from build123d import *

# Parameters (mm, degrees)
SKETCH009_W     = 7.72
SKETCH009_H     = 1
POCKET001_DEPTH = 26
POCKET002_DEPTH = 25


with BuildPart() as part:
    # Sketch008 → Revolution (revolve)
    with BuildSketch(Plane.XZ):
        Polygon((-1, 0), (-1, 3), (0, 3), (0, 2.5), (18.5, 2.5), (18.5, 3.2), (19.5, 2), (19.5, 0), align=None)
    revolve(axis=Axis((0, 0, 0), (1, 0, 0)))

    # Sketch009 → Pocket001 (cut)
    with BuildSketch(Plane.YZ):
        Rectangle(SKETCH009_W, SKETCH009_H)
    extrude(amount=POCKET001_DEPTH, mode=Mode.SUBTRACT)

    # Sketch010 → Pocket002 (cut, symmetric)
    with BuildSketch(Plane.XY):
        Polygon((15.1, 2.44949), (23.12, 2.44949), (23.12, -2.44949), (15.1, -2.44949), (15.1, -3.86051), (30.32, -3.86051), (30.32, 7.01949), (15.1, 7.01949), align=None)
    extrude(amount=POCKET002_DEPTH, both=True, mode=Mode.SUBTRACT)


with BuildPart() as part_1:
    # Body002 placement: moved
    add(part.part.moved(Location((-9.25, -10.5, 11.5))))


solid = part_1.part
Part model, mm, in its own coordinate system. A direction names the side the tool comes from. Round coordinates to 2 decimals unless told otherwise and drop trailing zeros. Order: outer loops, then holes, each group sorted by start corner. A loop starts at its lowest first (then second) coordinate and runs counter-clockwise, first axis right, second up. Notation, with made-up numbers: (-14.75, -19.75) -> (-10.75, -19.75) arc R33 ccw to (-10.75, 13.25) -> close; hole circle Ø1 at (-5, -13). An arc over 180 degrees is marked (long way). Put each result on its own line as item: value.
Q1. Band-saw the part on B-B (x = -7). Give the cut face in (y, z).
From the geometry:
outline: (-12.95, 11) arc R2.5 ccw to (-8.05, 11) -> close; (-12.95, 12) -> (-8.05, 12) arc R2.5 ccw to start
Q2. Band-saw the part on A-A (y = -10.5). Give the cut face in (x, z).
From the geometry:
outline: (-10.25, 8.5) -> (-9.25, 8.5) -> (-9.25, 9) -> (9.25, 9) -> (9.25, 8.3) -> (10.25, 9.5) -> (10.25, 11) -> (-9.25, 11) -> (-9.25, 12) -> (10.25, 12) -> (10.25, 13.5) -> (9.25, 14.7) -> (9.25, 14) -> (-9.25, 14) -> (-9.25, 14.5) -> (-10.25, 14.5) -> close
Q3. Pin check, flat tips, straight feed: pin 1 Ø1 at (y, z) = (-8, 13.5) entering from -X; pin 2 Ø1.5 at (x, y) = (4.5, -9) entering from +Z; pin 3 Ø0.6 at (x, z) = (9.5, 12.5) entering from +Y; pin 4 Ø0.6 at (x, z) = (9.5, 13) entering from -Y. Stop position of each tip, or through.
From the geometry:
pin 1: stops at x = -10.25
pin 2: stops at z = 13.88
pin 3: stops at y = -8.05
pin 4: stops at y = -12.95
Q4. Tool access for faces 1 (the face through (-9.25, -10.7, 11.5)), 2 (the face through (-9.7, -8.7, 9.1)), 3 (the face through (9.25, -10.3, 8.8)), 4 (the face through (0, -11, 12)), 5 (the face through (9.25, -10.5, 14.2)): list every direction of +Z, -Z, +X, -X, +Y, -Y with a clear straight run to the whole face (end or side of a thin tool).
From the geometry:
face 1: none
face 2: -X
face 3: -Z
face 4: +X, +Y, -Y
face 5: +Z
Q5. Pull direction X, two halves, no side cores. Call faces 6 (the face through (0, -11, 11)), 7 (the face through (0.1, -10.5, 14)), 8 (the face through (10.25, -11, 10)), 9 (the face through (-10.25, -11, 12)): pulls with the +X half, pulls with the -X half, needs draft (parallel to the pull), parting line crosses it, or undercut.
From the geometry:
face 6: needs draft
face 7: undercut
face 8: pulls with the +X half
face 9: pulls with the -X half
Q6. Wall check: line 1 (Z direction, x = -5.5, y = -10.55); line 2 (X direction, y = -9.1, z = 11.5); line 3 (X direction, y = -11.75, z = 13.75). Give the ranges that are in metal, low to high. Write a range as [from, to].
From the geometry:
line 1: z = [9, 11], [12, 14]
line 2: x = [-10.25, -9.25]
line 3: x = [-10.25, -9.25], [9.25, 9.77]
Q7. Band-saw the part on C-C (z = 11.5). Give the cut face in (x, y), and give its area (3 significant figures).
From the geometry:
outline: (-10.25, -13.5) -> (-9.25, -13.5) -> (-9.25, -7.5) -> (-10.25, -7.5) -> close
area: 6.00 mm2
